```python
from build123d import *

# Parameters (mm, degrees)
BOSS_EXTRUDE1_DEPTH  = 29.5
BOSS_EXTRUDE2_DEPTH  = 29
SKETCH7_W            = 1
SKETCH7_H            = 1
BOSS_EXTRUDE3_DEPTH  = 2
FILLET1_R            = 0.75
FILLET2_R            = 0.2
FILLET1_OF_MIRROR1_R = 0.75
FILLET2_OF_MIRROR1_R = 0.2
FILLET3_R            = 0.1


with BuildPart() as part:
    # Sketch1 → Boss-Extrude1 (new body)
    with BuildSketch(Plane(origin=(0, 0, 0), x_dir=(0, 0, -1), z_dir=(1, 0, 0))):
        Polygon((0, 0), (0, 0.4), (52.7, 0.4), (52.7, -0.4), (52.284313725, -0.4), (52.284313725, 0), align=None)
    boss_extrude1 = extrude(amount=BOSS_EXTRUDE1_DEPTH)

    # Sketch5 → Boss-Extrude2 (add)
    with BuildSketch(Plane(origin=(29.5, 0, -29.5), x_dir=(0, 0, 1), z_dir=(-1, 0, 0))):
        Polygon((29.5, 0.4), (-23.2, 0.4), (-23.2, -0.4), (-24.3, -0.4), (-24.3, 1.2), (29.5, 1.2), align=None)
    boss_extrude2 = extrude(amount=BOSS_EXTRUDE2_DEPTH)

    # Fillet1
    fillet1_edges = [part.edges().sort_by_distance(p)[0] for p in [
        (15, 1.2, 0),
    ]]
    fillet(fillet1_edges, radius=FILLET1_R)

    # Fillet2
    fillet2_edges = [part.edges().sort_by_distance(p)[0] for p in [
        (14.75, -0.4, -52.284313725),
    ]]
    fillet(fillet2_edges, radius=FILLET2_R)


with BuildPart() as body_2:
    # Sketch7 → Boss-Extrude3 (new body)
    with BuildSketch(Plane(origin=(29.5, 0, 0), x_dir=(0, 0, -1), z_dir=(1, 0, 0))):
        with Locations((1.496141384, 1.7)):
            Rectangle(SKETCH7_W, SKETCH7_H)
    boss_extrude3 = extrude(amount=-BOSS_EXTRUDE3_DEPTH)


with BuildPart() as part_1:
    add(part.part)

    add(body_2.part)  # Mirror1 merges body 2
    # Mirror1: Boss-Extrude1, Boss-Extrude2, Boss-Extrude3 across plane
    add(boss_extrude1.mirror(Plane.ZY.offset(-29.5)))
    add(boss_extrude2.mirror(Plane.ZY.offset(-29.5)))
    add(boss_extrude3.mirror(Plane.ZY.offset(-29.5)))

    # Fillet1 of Mirror1
    fillet1_of_mirror1_edges = [part_1.edges().sort_by_distance(p)[0] for p in [
        (44, 1.2, 0),
    ]]
    fillet(fillet1_of_mirror1_edges, radius=FILLET1_OF_MIRROR1_R)

    # Fillet2 of Mirror1
    fillet2_of_mirror1_edges = [part_1.edges().sort_by_distance(p)[0] for p in [
        (44.25, -0.4, -52.284313725),
    ]]
    fillet(fillet2_of_mirror1_edges, radius=FILLET2_OF_MIRROR1_R)

    # Fillet3
    fillet3_edges = [part_1.edges().sort_by_distance(p)[0] for p in [
        (29.5, 1.2, -0.996141384),
        (29.5, 2.2, -0.996141384),
        (29.5, 2.2, -1.996141384),
        (29.5, 1.2, -1.996141384),
        (31.5, 1.2, -1.496141384),
        (31.5, 1.7, -1.996141384),
        (31.5, 2.2, -1.496141384),
        (31.5, 1.7, -0.996141384),
        (27.5, 1.2, -1.496141384),
        (27.5, 1.7, -0.996141384),
        (27.5, 2.2, -1.496141384),
        (27.5, 1.7, -1.996141384),
    ]]
    fillet(fillet3_edges, radius=FILLET3_R)


solid = part_1.part
```
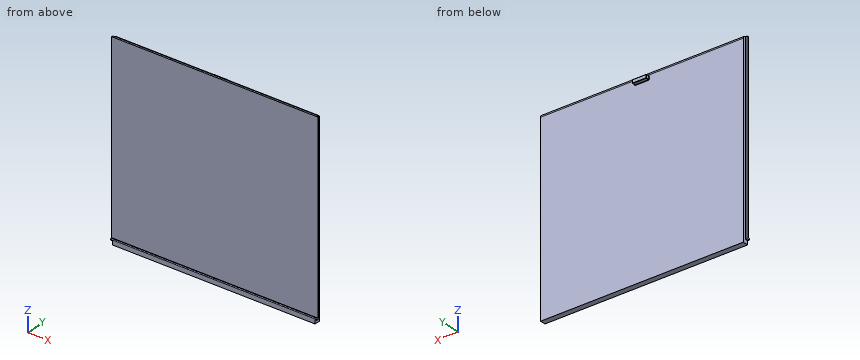
Here's how the part is built. I have some questions about the finished solid (model axes, mm). Give positions to 0.01 mm unless a question says otherwise; leave off trailing zeros. Write each loop counter-clockwise with the first axis right and the second up, starting at its lowest first coordinate (ties: lowest second). Pieces come first, ordered by that corner, then holes. Notation, with made-up numbers: M 25,33.25 L 45,33.25 A30 ccw 45,67.25 Z; hole C -2.5,57 d2. An arc over 180 degrees is marked long. Put each result on its own line as item: value. Start each with the question number.
Item 1: Will these pins go through, and if not, where does the flat tip stop? pin 1 (1 mm diameter, centred on y = 1, z = -41, fed in from +X); pin 2 (4 mm diameter, centred on x = 25, z = -9, fed in from +Y); pin 3 (3 mm diameter, centred on x = 49.5, z = -22.5, fed in from -Y).
Item 2: If we section it at C-C, the plane x = 30.5: Write out the boundary of the cut face in (y, z).
Item 3: If we section it at B-B, the plane y = 1.7: Write out the boundary of the cut face in (x, z).
Item 4: I need wall thicknesses on L1, parallel to Y at x = 8.5, z = -43.5; L2, parallel to Z at x = 33, y = 0.5. Which ranges of each line are inside material? Lowest first, please. Write a range as from..to.
Item 5: If we section it at A-A, the plane x = 42: Write out the boundary of the cut face in (y, z), then the cut area to 3 significant figures.
Values:
1. pin 1: x = 58.5
1. pin 2: y = 1.2
1. pin 3: y = 0
2. outline: M -0.4,-53.8 L 1.2,-53.8 L 1.2,-2.1 A0.1 cw 1.3,-2 L 2.1,-2 A0.1 ccw 2.2,-1.9 L 2.2,-1.1 A0.1 ccw 2.1,-1 L 1.3,-1 A0.1 cw 1.2,-0.9 L 1.2,-0.75 A0.75 ccw 0.45,0 L 0,0 L 0,-52.28 L -0.2,-52.28 A0.2 ccw -0.4,-52.48 Z
3. outline: M 27.5,-1.9 A0.1 ccw 27.6,-2 L 31.4,-2 A0.1 ccw 31.5,-1.9 L 31.5,-1.1 A0.1 ccw 31.4,-1 L 27.6,-1 A0.1 ccw 27.5,-1.1 Z
4. L1: 0..1.2
4. L2: -53.8..0
5. outline: M -0.4,-53.8 L 1.2,-53.8 L 1.2,-0.75 A0.75 ccw 0.45,0 L 0,0 L 0,-52.28 L -0.2,-52.28 A0.2 ccw -0.4,-52.48 Z
5. area: 65.0 mm²
